```python
from build123d import *

# Parameters (mm, degrees)
SKETCH1_R           = 1.27
SKETCH1_R_2         = 4.7625
SKETCH1_R_3         = 0.762
BOSS_EXTRUDE1_DEPTH = 3.048


with BuildPart() as part:
    # Sketch1 → Boss-Extrude1 (new body)
    with BuildSketch(Plane.XY):
        Polygon((552.957131224, 142.871693799), (562.737035343, 128.696327154), (512.803524332, 94.246075371), (503.023620213, 108.421442016), align=None)
        with Locations(Location((551.672296834, 136.012198904, 0), (0, 0, 180))):
            Circle(SKETCH1_R, mode=Mode.SUBTRACT)
        with Locations(Location((552.942296834, 128.696327154, 0), (0, 0, 180))):
            Circle(SKETCH1_R, mode=Mode.SUBTRACT)
        with Locations(Location((514.95104564, 106.189069777, 0), (0, 0, 180))):
            Circle(SKETCH1_R_2, mode=Mode.SUBTRACT)
        with Locations(Location((519.308599463, 115.367159158, 0), (0, 0, 180))):
            Circle(SKETCH1_R_3, mode=Mode.SUBTRACT)
        with Locations(Location((525.078281113, 107.004362159, 0), (0, 0, 180))):
            Circle(SKETCH1_R_3, mode=Mode.SUBTRACT)
    extrude(amount=BOSS_EXTRUDE1_DEPTH)


solid = part.part
```
Source: CAD feature listing. Evaluate the final solid. Frame: model axes, mm. Round coordinates to 2 decimals unless told otherwise and drop trailing zeros. Loops run counter-clockwise (first coordinate to the right, second up) from the corner with the lowest first, then second, coordinate; pieces in that order, holes last. Notation, with made-up numbers: M 40.5,81 L 78.5,81 A18 ccw 78.5,103 Z; hole C 49.5,10.5 d8. An arc over 180 degrees is marked long. Use a Markdown table: item, result. Add a question column.
1. Cut plane A-A, the plane z = 1.25. Output: boundary loops of the cut face in (x, y) (1 decimal), and give its area (3 significant figures).
2. Pull-direction query (Y, two-part tool) for faces 1 (the cylindrical face through (518.899, 114.725, 1.503)), 2 (the flat face through (535, 119, 3.048)), 3 (the flat face through (507.982, 101.235, 1.503)); classes: +Y half, -Y half, draft (parallel to the pull), parting line (faces both ways), or undercut.
3. Contact query for flat-ended pins moving along their axis: pin 1 (1.5 mm diameter, centred on y = 129.5, z = 0.5, fed in from +X); pin 2 (1.5 mm diameter, centred on x = 547, z = 2.5, fed in from +Y); pin 3 (1.5 mm diameter, centred on x = 551.67, y = 136.01, fed in from -Z). Output: stop coordinate, or through.
4. Ray query, line 1 along X through (y, z) = (106.5, 2.9); line 2 along X through (y, z) = (106, 0.5); line 3 along X through (y, z) = (116, 0.4). Return the intervals inside material, ascending. Write a range as [from, to].
5. Cut plane C-C, the plane y = 99. Output: boundary loops of the cut face in (x, z).
6. Cut plane B-B, the plane x = 533. Output: boundary loops of the cut face in (y, z), and give its area (3 significant figures).
Solution:
| question | item | result |
|---|---|---|
| 1 | outline | M 503,108.4 L 512.8,94.2 L 562.7,128.7 L 553,142.9 Z; hole C 515,106.2 d9.5; hole C 519.3,115.4 d1.5; hole C 525.1,107 d1.5; hole C 551.7,136 d2.5; hole C 552.9,128.7 d2.5 |
| 1 | area | 960 mm2 |
| 2 | face 1 | undercut |
| 2 | face 2 | draft |
| 2 | face 3 | -Y half |
| 3 | pin 1 | stops at x = 562.7 |
| 3 | pin 2 | stops at y = 139.28 |
| 3 | pin 3 | passes through |
| 4 | line 1 | x = [504.35, 510.2], [519.7, 524.51], [525.65, 530.56] |
| 4 | line 2 | x = [504.69, 510.19], [519.71, 529.84] |
| 4 | line 3 | x = [514.01, 518.88], [519.73, 544.33] |
| 5 | outline | M 509.52,0 L 519.69,0 L 519.69,3.05 L 509.52,3.05 Z |
| 6 | outline | M 108.18,0 L 129.1,0 L 129.1,3.05 L 108.18,3.05 Z |
| 6 | area | 63.8 mm2 |
